Source: CAD feature listing. Evaluate the final solid. Frame: model axes, mm. A direction names the side the tool comes from. Coordinates: 2 decimals unless noted, no trailing zeros. Order: outer loops, then holes, each group sorted by start corner. A loop starts at its lowest first (then second) coordinate and runs counter-clockwise, first axis right, second up. Notation, with made-up numbers: (-37.5, 35) - (-9.5, 35) arc R25 ccw to (-9.5, 73) - close; hole circle Ø9 at (43, 80.5). An arc over 180 degrees is marked (long way). One line per question, with ' | ' between items.
from build123d import *

# Parameters (mm, degrees)
F0_R     = 2.5
F1_DEPTH = 3
F3_DEPTH = 6
F4_R     = 2.5
F5_DEPTH = 3


with BuildPart() as f1:
    # F0 (on Top) → F1 (new body)
    with BuildSketch(Plane.XY):
        with BuildLine():
            ThreePointArc((-6.5, 5.95), (-12.45, 0), (-6.5, -5.95))
            Line((-6.5, -5.95), (6.5, -5.95))
            ThreePointArc((6.5, -5.95), (12.45, 0), (6.5, 5.95))
            Line((6.5, 5.95), (-6.5, 5.95))
        make_face()
        with Locations((-3.95, 0)):
            Circle(F0_R, mode=Mode.SUBTRACT)
        with Locations((-3.95, 0)):
            Circle(F0_R)
    extrude(amount=F1_DEPTH)

    # F2 (on face) → F3 (join)
    with BuildSketch(Plane.XY.offset(3)):
        with BuildLine():
            Line((6.5, 5.95), (0.55, 5.95))
            Line((0.55, 5.95), (0.55, -5.95))
            Line((0.55, -5.95), (6.5, -5.95))
            ThreePointArc((6.5, -5.95), (12.45, 0), (6.5, 5.95))
        make_face()
    extrude(amount=F3_DEPTH)

    # F4 (on face) → F5 (cut)
    with BuildSketch(Plane.XY.offset(3)):
        with Locations((-3.95, 0)):
            Circle(F4_R)
    extrude(amount=-F5_DEPTH, mode=Mode.SUBTRACT)


solid = f1.part
(1) Cut plane C-C (z = 2.75). Return the cut outline in (x, y).
Taken from the geometry:
outline: (-6.5, -5.95) - (6.5, -5.95) arc R5.95 ccw to (6.5, 5.95) - (-6.5, 5.95) arc R5.95 ccw to start; hole circle Ø5 at (-3.95, 0)
(2) Pin query (flat end, axial travel): P1, Ø4, axis at y = -4, z = 2, coming from the -X side; P2, Ø6, axis at x = -6, y = -2.5, coming from the +Z side; P3, Ø3, axis at y = -1, z = 5.5, coming from the -X side. Return the tip coordinate at first contact, or that it passes through.
Taken from the geometry:
P1: stops at x = -12.1 | P2: stops at z = 3 | P3: stops at x = 0.55
(3) Cut plane A-A (x = -3.95). Return the cut outline in (y, z).
Taken from the geometry:
outline: (-5.95, 0) - (-2.5, 0) - (-2.5, 3) - (-5.95, 3) - close; (2.5, 0) - (5.95, 0) - (5.95, 3) - (2.5, 3) - close
(4) Set-up query: faces 1 (the cylindrical face through (-5.934, -1.521, 1.521)), 2 (the flat face through (0.55, 0, 6)). Return all of +Z, -Z, +X, -X, +Y, -Y with unobstructed straight access to the full face (end or side cutting, diameter ignored); none if empty.
Taken from the geometry:
face 1: +Z, -Z | face 2: +Z, -X, +Y, -Y
(5) Cut plane D-D (y = -2.25). Return the cut outline in (x, z).
Taken from the geometry:
outline: (-12.01, 0) - (-5.04, 0) - (-5.04, 3) - (-12.01, 3) - close; (-2.86, 0) - (12.01, 0) - (12.01, 9) - (0.55, 9) - (0.55, 3) - (-2.86, 3) - close
(6) Cut plane B-B (y = 0). Return the cut outline in (x, z), and give its area (3 significant figures).
Taken from the geometry:
outline: (-12.45, 0) - (-6.45, 0) - (-6.45, 3) - (-12.45, 3) - close; (-1.45, 0) - (12.45, 0) - (12.45, 9) - (0.55, 9) - (0.55, 3) - (-1.45, 3) - close | area: 131 mm²
(7) Material intervals for L1, parallel to Y at x = -3.95, z = 0.65; L2, parallel to Z at x = -9.25, y = -4.5; L3, parallel to Y at x = 9, z = 0.5, sorted ascending. Write a range as from..to.
Taken from the geometry:
L1: y = -5.95..-2.5, 2.5..5.95 | L2: z = 0..3 | L3: y = -5.4..5.4
